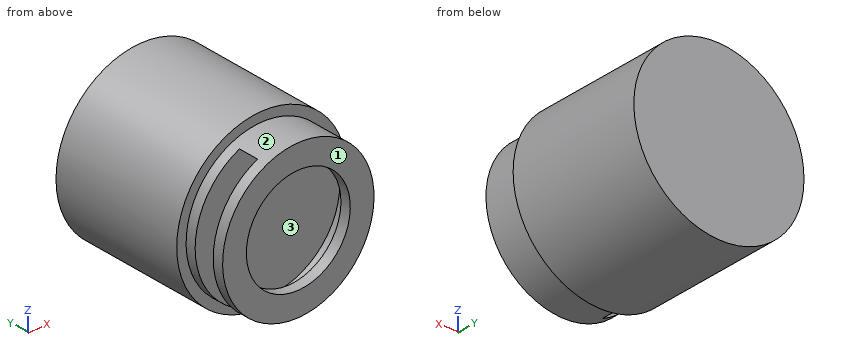
```python
from build123d import *

# Parameters (mm, degrees)
SKETCH5_R           = 22.25
SKETCH5_R_2         = 15.275
BOSS_EXTRUDE1_DEPTH = 3.1
SKETCH6_R           = 22.25
SKETCH6_R_2         = 20.25
BOSS_EXTRUDE2_DEPTH = 6
SKETCH7_R           = 22.25
BOSS_EXTRUDE3_DEPTH = 3
SKETCH8_R           = 25
BOSS_EXTRUDE4_DEPTH = 40
SKETCH9_W           = 22.25
SKETCH9_H           = 40.5
CUT_EXTRUDE1_DEPTH  = 6


with BuildPart() as part:
    # Sketch5 → Boss-Extrude1 (new body)
    with BuildSketch(Plane(origin=(0, 0, 0), x_dir=(1, 0, 0), z_dir=(0, 1, 0))):
        with Locations(Location((0, 0, 0), (0, 0, 90))):
            Circle(SKETCH5_R)
        with Locations(Location((0, 0, 0), (0, 0, 90))):
            Circle(SKETCH5_R_2, mode=Mode.SUBTRACT)
    extrude(amount=BOSS_EXTRUDE1_DEPTH)

    # Sketch6 → Boss-Extrude2 (add)
    with BuildSketch(Plane(origin=(0, 3.1, 0), x_dir=(1, 0, 0), z_dir=(0, 1, 0))):
        with Locations(Location((0, 0, 0), (0, 0, 90))):
            Circle(SKETCH6_R)
        with Locations(Location((0, 0, 0), (0, 0, 270))):
            Circle(SKETCH6_R_2, mode=Mode.SUBTRACT)
    extrude(amount=BOSS_EXTRUDE2_DEPTH)

    # Sketch7 → Boss-Extrude3 (add)
    with BuildSketch(Plane(origin=(0, 9.1, 0), x_dir=(1, 0, 0), z_dir=(0, 1, 0))):
        with Locations(Location((0, 0, 0), (0, 0, 90))):
            Circle(SKETCH7_R)
    extrude(amount=BOSS_EXTRUDE3_DEPTH)

    # Sketch8 → Boss-Extrude4 (add)
    with BuildSketch(Plane(origin=(0, 12.1, 0), x_dir=(1, 0, 0), z_dir=(0, 1, 0))):
        with Locations(Location((0, 0, 0), (0, 0, 270))):
            Circle(SKETCH8_R)
    extrude(amount=BOSS_EXTRUDE4_DEPTH)

    # Sketch9 → Cut-Extrude1 (cut)
    with BuildSketch(Plane(origin=(0, 3.1, 0), x_dir=(1, 0, 0), z_dir=(0, 1, 0))):
        with Locations((-11.125, 0)):
            Rectangle(SKETCH9_W, SKETCH9_H)
    extrude(amount=CUT_EXTRUDE1_DEPTH, mode=Mode.SUBTRACT)


solid = part.part
```
Design review of the part built by this model. Coordinates are the model's own, in mm. Face numbers are marked on the shaded views. Coordinates: 2 decimals unless noted, no trailing zeros. Order: outer loops, then holes, each group sorted by start corner. A loop starts at its lowest first (then second) coordinate and runs counter-clockwise, first axis right, second up. Notation, with made-up numbers: (7, 5.25) -> (39, 5.25) arc R22 cw to (39, 38.25) -> close; hole circle Ø11 at (-21.5, 10.25). An arc over 180 degrees is marked (long way). One line per item, written item: value. Start each with the question number.
Q1. Take a section at A-A, the plane z = 0. State the section outline as (x, y) points (3 decimals), then the cut area to 3 significant figures.
Q2. Take a section at B-B, the plane x = -12. State the section outline as (y, z) points.
Q3. Take a section at C-C, the plane y = 44. State the section outline as (x, z) points, then the cut area to 3 significant figures.
Q4. For probe 1 along Y at (x, z) = (0.5, 16); probe 2 along X at (y, z) = (1.8, 0) (3 decimals); probe 3 along Y at (x, z) = (-9.5, 9.5), list the stretches that pass through material, from the lowest coordinate up.
Q5. Mouldability with a two-part tool opening along Z and no side actions: class the marked faces 1, 2 and 3 as pulls with the +Z half, pulls with the -Z half, needs draft (parallel to the pull), parting line crosses it, or undercut.
Q6. Take a section at D-D, the plane z = 12. State the section outline as (x, y) points, then the cut area to 3 significant figures.
Q7. Insertion check: pin 1 Ø8 at (y, z) = (26, -11) entering from +X; pin 2 Ø12 at (x, y) = (16, 5.5) entering from -Z; pin 3 Ø3 at (x, y) = (-4, 5.5) entering from +Z. Each pin has a flat end and moves straight along its axis. Give the tip position at first contact, or say it passes through.
Values follow:
1. outline: (-25, 12.1) -> (-22.25, 12.1) -> (-22.25, 9.1) -> (20.25, 9.1) -> (20.25, 3.1) -> (15.275, 3.1) -> (15.275, 0) -> (22.25, 0) -> (22.25, 12.1) -> (25, 12.1) -> (25, 52.1) -> (-25, 52.1) -> close; (-22.25, 0) -> (-15.275, 0) -> (-15.275, 3.1) -> (-22.25, 3.1) -> close
1. area: 2,190 mm2
2. outline: (0, -18.74) -> (3.1, -18.74) -> (3.1, -9.45) -> (0, -9.45) -> close; (0, 9.45) -> (3.1, 9.45) -> (3.1, 18.74) -> (0, 18.74) -> close; (9.1, -18.74) -> (12.1, -18.74) -> (12.1, -21.93) -> (52.1, -21.93) -> (52.1, 21.93) -> (12.1, 21.93) -> (12.1, 18.74) -> (9.1, 18.74) -> close
3. outline: circle Ø50 at (0, 0)
3. area: 1,960 mm2
4. probe 1: y = 0 to 3.1, 9.1 to 52.1
4. probe 2: x = -22.25 to -15.275, 15.275 to 22.25
4. probe 3: y = 9.1 to 52.1
5. face 1: needs draft
5. face 2: parting line crosses it
5. face 3: undercut
6. outline: (-21.93, 12.1) -> (-18.74, 12.1) -> (-18.74, 9.1) -> (16.31, 9.1) -> (16.31, 3.1) -> (9.45, 3.1) -> (9.45, 0) -> (18.74, 0) -> (18.74, 12.1) -> (21.93, 12.1) -> (21.93, 52.1) -> (-21.93, 52.1) -> close; (-18.74, 0) -> (-9.45, 0) -> (-9.45, 3.1) -> (-18.74, 3.1) -> close
6. area: 1,940 mm2
7. pin 1: stops at x = 24
7. pin 2: stops at z = -19.88
7. pin 3: stops at z = 22.11
